Autodesk Inventor part; units mm, degrees
ref_plane "YZ Plane" through (0, 0, 0) normal (1, 0, 0) x (0, 1, 0)
ref_plane "XZ Plane" through (0, 0, 0) normal (0, 1, 0) x (-1, 0, 0)
ref_plane "XY Plane" through (0, 0, 0) normal (0, 0, 1) x (1, 0, 0)
sketch "Sketch1" plane through (0, 0, 0) normal (0, 1, 0) x (-1, 0, 0)
  line L0 (-8.25, 14.464) -> (8.25, 14.464) construction
  line L1 (8.25, 14.464) -> (8.25, -14.464) construction
  line L2 (8.25, -14.464) -> (-8.25, -14.464) construction
  line L3 (-8.25, -14.464) -> (-8.25, 14.464) construction
  line L4 (-8.25, 14.464) -> (8.25, -14.464) construction
  line L5 (8.25, 14.464) -> (-8.25, -14.464) construction
  circle A0 centre (8.25, 14.464) radius 1
  circle A1 centre (8.25, -14.464) radius 1
  circle A2 centre (-8.25, -14.464) radius 1
  circle A3 centre (-8.25, 14.464) radius 1
  line L6 (-4.3, 3.55) -> (4.3, 3.55)
  line L7 (4.3, 3.55) -> (4.3, -3.55)
  line L8 (4.3, -3.55) -> (-4.3, -3.55)
  line L9 (-4.3, -3.55) -> (-4.3, 3.55)
  line L10 (-4.3, 3.55) -> (4.3, -3.55) construction
  line L11 (4.3, 3.55) -> (-4.3, -3.55) construction
  circle A4 centre (8.25, 14.464) radius 2
  circle A5 centre (8.25, -14.464) radius 2
  circle A6 centre (-8.25, -14.464) radius 2
  circle A7 centre (-8.25, 14.464) radius 2
  arc A8 (10.1962, 14.0034) -> (10.1962, -14.0034) centre (69.3616, 0) ccw
  arc A9 (-10.1962, -14.0034) -> (-10.1962, 14.0034) centre (-69.3616, 0) ccw
  arc A10 (7.8571, -16.425) -> (-7.8571, -16.425) centre (0, -55.6458) ccw
  arc A11 (-7.8571, 16.425) -> (7.8571, 16.425) centre (0, 55.6458) ccw
  point P0 (0, 0)
  dimension "d0" = 16.5
  dimension "d1" = 28.928
  dimension "d2" = 2
  dimension "d3" = 2
  dimension "d4" = 2
  dimension "d5" = 2
  dimension "d6" = 8.6
  dimension "d7" = 7.1
  dimension "d8" = 4
  dimension "d9" = 4
  dimension "d10" = 4
  dimension "d11" = 4
  dimension "d12" = 60.8
  dimension "d13" = 60.8
  dimension "d14" = 40
  dimension "d15" = 40
extrude "Extrusion1" add sketch "Sketch1" along normal blind 3
properties part number "Seal_plate"
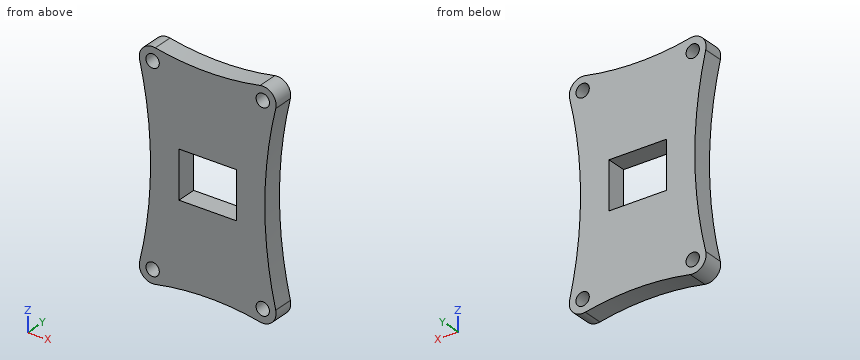
Here's how the part is built. I have some questions about the finished solid (model axes, mm). Give positions to 0.01 mm unless a question says otherwise; leave off trailing zeros. Order: outer loops, then holes, each group sorted by start corner. A loop starts at its lowest first (then second) coordinate and runs counter-clockwise, first axis right, second up. Notation, with made-up numbers: (-34.75, -6.75) - (-23.75, -6.75) arc R12 cw to (-23.75, 4.25) - close; hole circle Ø10 at (-15, -26.75). An arc over 180 degrees is marked (long way). Answer as a JSON object with one key per item and string values. Group by question number.
Item 1: Please list where these lines run through material, in increasing order: probe 1 along Z at (x, y) = (8.25, 1.5); probe 2 along X at (y, z) = (1.85, 14.5); probe 3 along X at (y, z) = (1.8, 1).
Item 2: If we section it at B-B on x = -3: Please give me the cut outline in (y, z), and give its area (3 significant figures).
Item 3: If we section it at A-A on x = -8.25: Please give me the cut outline in (y, z).
Item 4: If we section it at D-D on y = 0.6: Please give me the cut outline in (x, z) (3 decimals), and give its area (3 significant figures).
Item 5: If we section it at C-C on z = -1: Please give me the cut outline in (x, y), and give its area (3 significant figures).
Item 6: For P1, Ø1.5, axis at x = -2.5, y = 1, coming from the +Z side; P2, Ø1.2, axis at x = -8.25, z = 14.464, coming from the -Y side; P3, Ø1, axis at x = 2, y = 2, coming from the -Z side; P4, Ø1.5, axis at y = 0.5, z = -1, coming from the -X side, each with a flat end and sliding along its axis, tell me the tip position at first contact or that it passes through.
Result set:
{
 "1": {"probe 1": "-16.46 to -15.46, -13.46 to 13.46, 15.46 to 16.46", "probe 2": "-10.25 to -9.25, -7.25 to 7.25, 9.25 to 10.25", "probe 3": "-8.57 to -4.3, 4.3 to 8.57"},
 "2": {"outline": "(0, -15.76) - (3, -15.76) - (3, -3.55) - (0, -3.55) - close; (0, 3.55) - (3, 3.55) - (3, 15.76) - (0, 15.76) - close", "area": "73.3 mm²"},
 "3": {"outline": "(0, -16.46) - (3, -16.46) - (3, -15.46) - (0, -15.46) - close; (0, -13.46) - (3, -13.46) - (3, 13.46) - (0, 13.46) - close; (0, 15.46) - (3, 15.46) - (3, 16.46) - (0, 16.46) - close"},
 "4": {"outline": "(-10.196, -14.003) arc R2 ccw to (-7.857, -16.425) arc R40 cw to (7.857, -16.425) arc R2 ccw to (10.196, -14.003) arc R60.8 cw to (10.196, 14.003) arc R2 ccw to (7.857, 16.425) arc R40 cw to (-7.857, 16.425) arc R2 ccw to (-10.196, 14.003) arc R60.8 cw to start; hole circle Ø2 at (-8.25, -14.464); hole circle Ø2 at (-8.25, 14.464); hole (-4.3, -3.55) - (4.3, -3.55) - (4.3, 3.55) - (-4.3, 3.55) - close; hole circle Ø2 at (8.25, -14.464); hole circle Ø2 at (8.25, 14.464)", "area": "516 mm²"},
 "5": {"outline": "(-8.57, 0) - (-4.3, 0) - (-4.3, 3) - (-8.57, 3) - close; (4.3, 0) - (8.57, 0) - (8.57, 3) - (4.3, 3) - close", "area": "25.6 mm²"},
 "6": {"P1": "z = 15.78", "P2": "through", "P3": "z = -15.72", "P4": "x = -8.59"}
}
